Autodesk Inventor part; units mm, degrees
ref_plane "to_block_XY" through (0, 5.5, 0) normal (0, 0, 1) x (1, 0, 0)
ref_plane "to_block_YZ" through (0, 5.5, 0) normal (1, 0, 0) x (0, 1, 0)
ref_plane "to_block_ZX" through (0, 5.5, 0) normal (0, 1, 0) x (0, 0, 1)
sketch "Sketch_12" plane through (0, 0, 0) normal (0, 0, 1) x (1, 0, 0)
  line L0 (-4.5, 5.3) -> (-4.5, 5.0434)
  line L1 (-4.5, 5.0434) -> (-4.2216, 4.8827)
  arc A0 (-3.7548, 4.35) -> (-4.2216, 4.8827) centre (-4.7715, 3.93) ccw
  line L2 (-3.7548, 4.35) -> (-3.1, 4.35)
  line L3 (-3.1, 4.35) -> (-3.1, 3.65)
  line L4 (-3.1, 3.65) -> (-3.7548, 3.65)
  arc A1 (-4.2216, 3.1173) -> (-3.7548, 3.65) centre (-4.7715, 4.07) ccw
  line L5 (-4.2216, 3.1173) -> (-4.5, 2.9566)
  line L6 (-4.5, 2.9566) -> (-4.5, 0.3)
  line L7 (-4.5, 0.3) -> (-4.2, 0)
  line L8 (-4.2, 0) -> (4.2, 0)
  line L9 (4.2, 0) -> (4.5, 0.3)
  line L10 (4.5, 0.3) -> (4.5, 2.9566)
  line L11 (4.5, 2.9566) -> (4.2216, 3.1173)
  arc A2 (3.7548, 3.65) -> (4.2216, 3.1173) centre (4.7715, 4.07) ccw
  line L12 (3.7548, 3.65) -> (3.1, 3.65)
  line L13 (3.1, 3.65) -> (3.1, 4.35)
  line L14 (3.1, 4.35) -> (3.7548, 4.35)
  arc A3 (4.2216, 4.8827) -> (3.7548, 4.35) centre (4.7715, 3.93) ccw
  line L15 (4.2216, 4.8827) -> (4.5, 5.0434)
  line L16 (4.5, 5.0434) -> (4.5, 5.3)
  line L17 (4.5, 5.3) -> (4.3, 5.5)
  line L18 (4.3, 5.5) -> (-4.3, 5.5)
  line L19 (-4.3, 5.5) -> (-4.5, 5.3)
extrude "Extrusion1" add sketch "Sketch_12" along normal mid plane 55
sketch "Sketch2" plane through (-4.3, 5.5, 27.5) normal (0, 1, 0) x (1, 0, 0)
  point P0 (4.3, 47.5)
hole "Hole1" at (0, 5.5, -20) direction (0, -1, 0) diameter 3.5 depth 5.5 counterbore diameter 6 counterbore depth 3.5
pattern_linear "Rectangular Pattern1" count 3 spacing 20 along (0, 0, 1) of "Hole1"
ref_plane "to_block_XY" through (0, 5.5, 0) normal (0, 0, 1) x (1, 0, 0)
ref_plane "to_block_YZ" through (0, 5.5, 0) normal (1, 0, 0) x (0, 1, 0)
ref_plane "to_block_ZX" through (0, 5.5, 0) normal (0, 1, 0) x (0, 0, 1)
properties part number "SSEBZ-MX10-55_r"
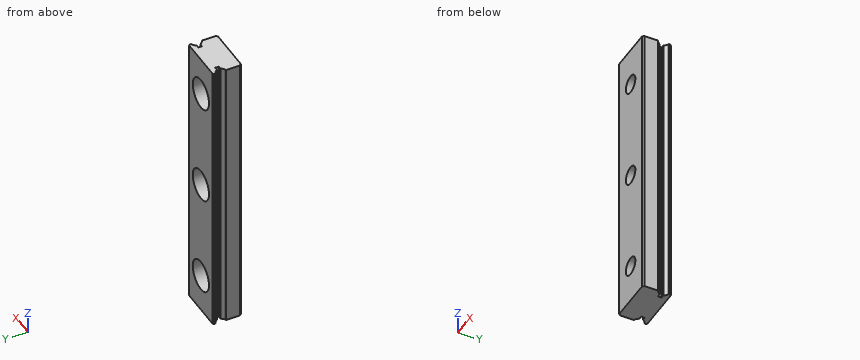
Check sheet for the modelled part. Datum: model origin and axes. Units: mm. Give positions to 0.01 mm unless a question says otherwise; leave off trailing zeros. Order: outer loops, then holes, each group sorted by start corner. A loop starts at its lowest first (then second) coordinate and runs counter-clockwise, first axis right, second up. Notation, with made-up numbers: M 21,57.25 L 58,57.25 A6 cw 58,66.25 Z; hole C 40.5,4 d10. An arc over 180 degrees is marked long. Answer in a Markdown table with one row per item.
1) Cross-section at C-C, the plane y = 1.1. Enter the section's corners in (x, z), plus the area to 3 significant figures.
Filled sheet:
| item | result |
|---|---|
| outline | M -4.5,-27.5 L 4.5,-27.5 L 4.5,27.5 L -4.5,27.5 Z; hole C 0,-20 d3.5; hole C 0,0 d3.5; hole C 0,20 d3.5 |
| area | 466 mm2 |
2) Cross-section at D-D, the plane z = -8. Enter the section's corners in (x, y).
Filled sheet:
| item | result |
|---|---|
| outline | M -4.5,0.3 L -4.2,0 L 4.2,0 L 4.5,0.3 L 4.5,2.96 L 4.22,3.12 A1.1 cw 3.75,3.65 L 3.1,3.65 L 3.1,4.35 L 3.75,4.35 A1.1 cw 4.22,4.88 L 4.5,5.04 L 4.5,5.3 L 4.3,5.5 L -4.3,5.5 L -4.5,5.3 L -4.5,5.04 L -4.22,4.88 A1.1 cw -3.75,4.35 L -3.1,4.35 L -3.1,3.65 L -3.75,3.65 A1.1 cw -4.22,3.12 L -4.5,2.96 Z |
3) Gauge pin test, flat ends, axial feed: P1, Ø1, axis at y = 4, z = 0, coming from the +X side; P2, Ø4, axis at x = 1, z = 2, coming from the +Y side; P3, Ø1.8, axis at x = 1.5, z = -19.5, coming from the +Y side; P4, Ø0.6, axis at y = 4, z = -3, coming from the -X side. Record the tip position at first contact, or that the pin passes through.
Filled sheet:
| item | result |
|---|---|
| P1 | stops at x = 3.83 |
| P2 | stops at y = 5.5 |
| P3 | stops at y = 2 |
| P4 | stops at x = -3.1 |
4) Cross-section at B-B, the plane x = 0. Enter the section's corners in (y, z), plus the area to 4 significant figures.
Filled sheet:
| item | result |
|---|---|
| outline | M 0,-27.5 L 5.5,-27.5 L 5.5,-23 L 2,-23 L 2,-21.75 L 0,-21.75 Z; M 0,-18.25 L 2,-18.25 L 2,-17 L 5.5,-17 L 5.5,-3 L 2,-3 L 2,-1.75 L 0,-1.75 Z; M 0,1.75 L 2,1.75 L 2,3 L 5.5,3 L 5.5,17 L 2,17 L 2,18.25 L 0,18.25 Z; M 0,21.75 L 2,21.75 L 2,23 L 5.5,23 L 5.5,27.5 L 0,27.5 Z |
| area | 218.5 mm2 |
5) Thickness scan on L1, parallel to Z at x = 0, y = 1.4; L2, parallel to Z at x = 0, y = 4.25; L3, parallel to X at y = 0.9, z = 20. Record the ranges inside material, lowest first. Write a range as [from, to].
Filled sheet:
| item | result |
|---|---|
| L1 | z = [-27.5, -21.75], [-18.25, -1.75], [1.75, 18.25], [21.75, 27.5] |
| L2 | z = [-27.5, -23], [-17, -3], [3, 17], [23, 27.5] |
| L3 | x = [-4.5, -1.75], [1.75, 4.5] |
